The drawing under review shows one solid part. Ordinate dimensions are in mm from its lowest x, y, z. A direction names the side the tool comes from. Round coordinates to 2 decimals unless told otherwise and drop trailing zeros. Write each loop counter-clockwise with the first axis right and the second up, starting at its lowest first coordinate (ties: lowest second). Pieces come first, ordered by that corner, then holes. Notation, with made-up numbers: (-34.5, -13.5) -> (-6.5, -13.5) arc R21 ccw to (-6.5, -7.5) -> close; hole circle Ø9 at (30, 50.5). An arc over 180 degrees is marked (long way). Answer in a Markdown table with one row per item.
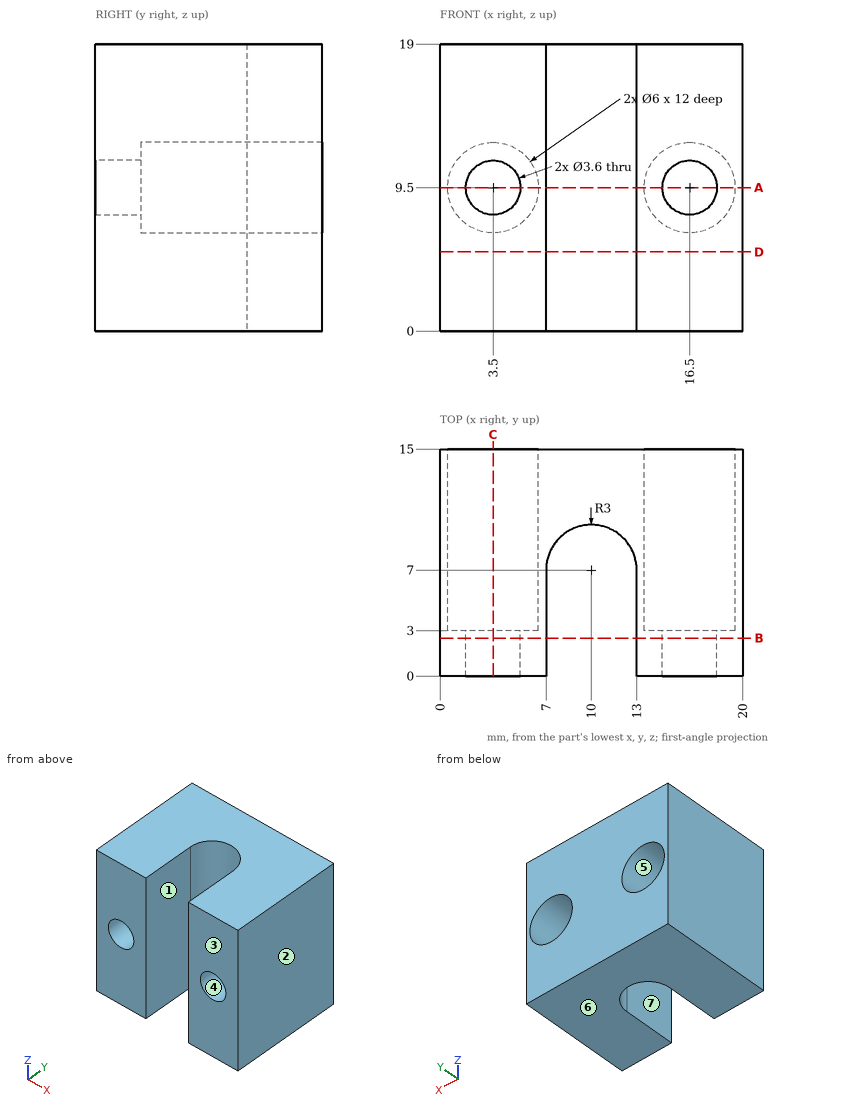
1) Clearance check with flat-ended pins moving along their axes: pin 1 Ø4 at (x, z) = (16.5, 9.5) entering from +Y; pin 2 Ø1 at (x, z) = (8.5, 14.5) entering from -Y. State where each tip first meets the part, or that it passes through.
Solved:
| item | result |
|---|---|
| pin 1 | y = 3 |
| pin 2 | y = 9.24 |
2) For the marked faces 5, 6 and 7, list the 3-axis set-ups (+Z, -Z, +X, -X, +Y, -Y) from which the entire face can be reached by the end or side of a thin tool; tool diameter is ignored.
Solved:
| item | result |
|---|---|
| face 5 | +Y |
| face 6 | -Z, +X, -X, +Y, -Y |
| face 7 | +Z, -Z, -Y |
3) Consider section D-D on z = 5.25. State the section outline as (x, y) points, then the cut area to 3 significant figures.
Solved:
| item | result |
|---|---|
| outline | (0, 0) -> (7, 0) -> (7, 7) arc R3 cw to (13, 7) -> (13, 0) -> (20, 0) -> (20, 15) -> (0, 15) -> close |
| area | 244 mm² |
4) Mouldability with a two-part tool opening along X and no side actions: class the marked faces 1, 2, 3 and 4 as pulls with the +X half, pulls with the -X half, needs draft (parallel to the pull), parting line crosses it, or undercut.
Solved:
| item | result |
|---|---|
| face 1 | undercut |
| face 2 | pulls with the +X half |
| face 3 | needs draft |
| face 4 | undercut |
5) Consider section B-B on y = 2.5. State the section outline as (x, z) points.
Solved:
| item | result |
|---|---|
| outline | (0, 0) -> (7, 0) -> (7, 19) -> (0, 19) -> close; (13, 0) -> (20, 0) -> (20, 19) -> (13, 19) -> close; hole circle Ø3.6 at (3.5, 9.5); hole circle Ø3.6 at (16.5, 9.5) |
6) Consider section C-C on x = 3.5. State the section outline as (y, z) points, then the cut area to 3 significant figures.
Solved:
| item | result |
|---|---|
| outline | (0, 0) -> (15, 0) -> (15, 6.5) -> (3, 6.5) -> (3, 7.7) -> (0, 7.7) -> close; (0, 11.3) -> (3, 11.3) -> (3, 12.5) -> (15, 12.5) -> (15, 19) -> (0, 19) -> close |
| area | 202 mm² |
7) Consider section A-A on z = 9.5. State the section outline as (x, y) points, then the cut area to 3 significant figures.
Solved:
| item | result |
|---|---|
| outline | (0, 0) -> (1.7, 0) -> (1.7, 3) -> (0.5, 3) -> (0.5, 15) -> (0, 15) -> close; (5.3, 0) -> (7, 0) -> (7, 7) arc R3 cw to (13, 7) -> (13, 0) -> (14.7, 0) -> (14.7, 3) -> (13.5, 3) -> (13.5, 15) -> (6.5, 15) -> (6.5, 3) -> (5.3, 3) -> close; (18.3, 0) -> (20, 0) -> (20, 15) -> (19.5, 15) -> (19.5, 3) -> (18.3, 3) -> close |
| area | 78.3 mm² |
8) For line 1 (X direction, y = 12.25, z = 9.5); line 2 (X direction, y = 2.2, z = 9.5); line 3 (X direction, y = 5.5, z = 17), list the stretches that pass through material, from the lowest coordinate up. Write a range as [from, to].
Solved:
| item | result |
|---|---|
| line 1 | [0, 0.5], [6.5, 13.5], [19.5, 20] |
| line 2 | [0, 1.7], [5.3, 7], [13, 14.7], [18.3, 20] |
| line 3 | [0, 7], [13, 20] |
